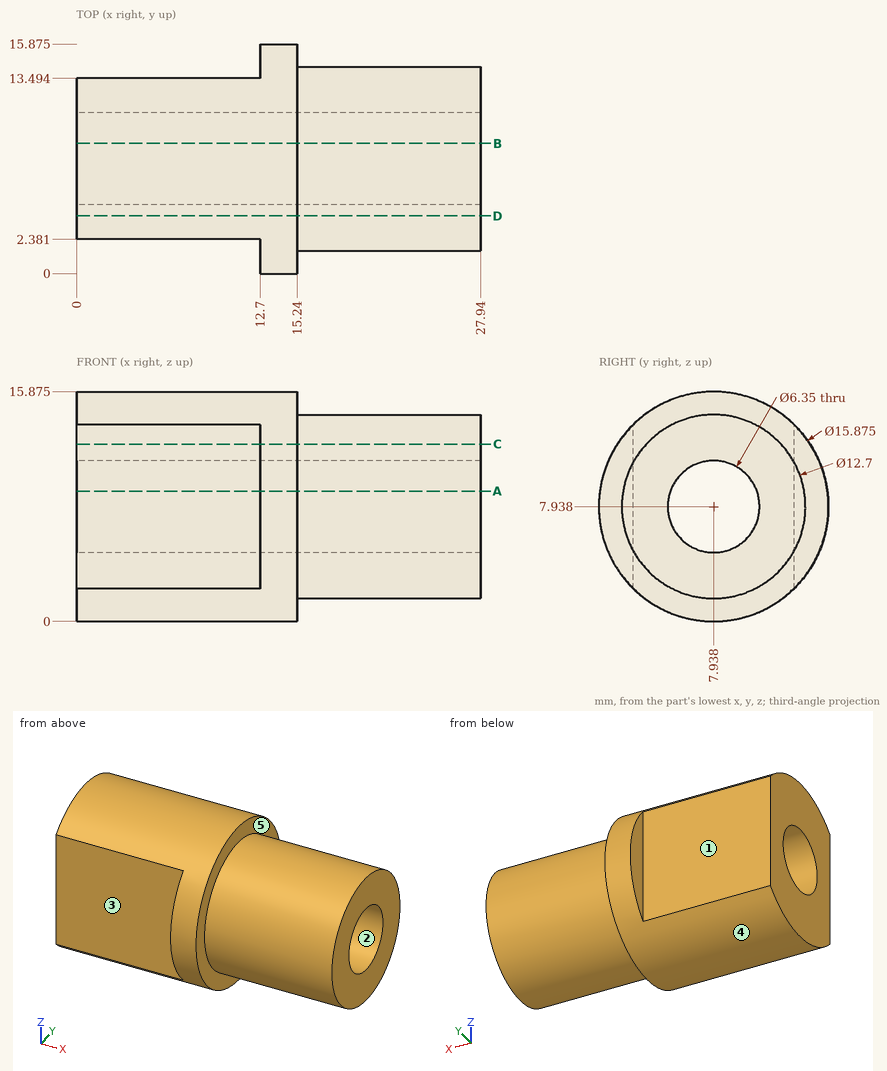
Print and shaded views of the part. All mm, measured from the part's lowest x, y and z. A direction names the side the tool comes from. Coordinates: 2 decimals unless noted, no trailing zeros. Order: outer loops, then holes, each group sorted by start corner. A loop starts at its lowest first (then second) coordinate and runs counter-clockwise, first axis right, second up.
(1) Tool access for the marked faces 4 and 5: list every direction of +Z, -Z, +X, -X, +Y, -Y with a clear straight run to the whole face (end or side of a thin tool).
Check sheet entries:
face 4: +X, -X
face 5: +X
(2) Pin check, flat tips, straight feed: pin 1 Ø5 at (y, z) = (11, 13.5) entering from -X; pin 2 Ø4 at (x, z) = (24, 5.5) entering from +Y; pin 3 Ø9 at (x, z) = (7, 9) entering from +Y; pin 4 Ø5 at (x, z) = (19, 14) entering from -Y. Stop position of each tip, or through.
Check sheet entries:
pin 1: stops at x = 0
pin 2: stops at y = 14.27
pin 3: stops at y = 13.49
pin 4: stops at y = 2.68
(3) Probe L1, parallel to X at y = 13.25, z = 13; L2, parallel to Y at x = 1, z = 11.5; L3, parallel to Z at x = 18.5, y = 7.75 (1 decimal). List the from-to ranges inside material, lowest first.
Check sheet entries:
L1: x = 0 to 15.24
L2: y = 2.38 to 13.49
L3: z = 1.6 to 4.8, 11.1 to 14.3
(4) Slice it at B-B, the plane y = 9. Write the cut outline in (x, z) (1 decimal).
Check sheet entries:
outline: (0, 0.1) - (15.2, 0.1) - (15.2, 1.7) - (27.9, 1.7) - (27.9, 4.9) - (0, 4.9) - close; (0, 10.9) - (27.9, 10.9) - (27.9, 14.2) - (15.2, 14.2) - (15.2, 15.8) - (0, 15.8) - close
(5) Slice it at A-A, the plane z = 9. Write the cut outline in (x, y) (1 decimal), and give its area (3 significant figures).
Check sheet entries:
outline: (0, 2.4) - (12.7, 2.4) - (12.7, 0.1) - (15.2, 0.1) - (15.2, 1.7) - (27.9, 1.7) - (27.9, 4.9) - (0, 4.9) - close; (0, 10.9) - (27.9, 10.9) - (27.9, 14.2) - (15.2, 14.2) - (15.2, 15.8) - (12.7, 15.8) - (12.7, 13.5) - (0, 13.5) - close
area: 173 mm2
(6) Slice it at D-D, the plane y = 4. Write the cut outline in (x, z) (1 decimal), and give its area (3 significant figures).
Check sheet entries:
outline: (0, 1) - (15.2, 1) - (15.2, 3) - (27.9, 3) - (27.9, 12.9) - (15.2, 12.9) - (15.2, 14.8) - (0, 14.8) - close
area: 337 mm2
(7) Slice it at C-C, the plane z = 12.25. Write the cut outline in (x, y), and give its area (3 significant figures).
Check sheet entries:
outline: (0, 2.38) - (12.7, 2.38) - (12.7, 1.27) - (15.24, 1.27) - (15.24, 3.28) - (27.94, 3.28) - (27.94, 12.6) - (15.24, 12.6) - (15.24, 14.6) - (12.7, 14.6) - (12.7, 13.49) - (0, 13.49) - close
area: 293 mm2
(8) Pull direction Y, two halves, no side cores. Call the marked faces 1, 2 and 3: pulls with the +Y half, pulls with the -Y half, needs draft (parallel to the pull), parting line crosses it, or undercut.
Check sheet entries:
face 1: pulls with the +Y half
face 2: undercut
face 3: pulls with the -Y half
